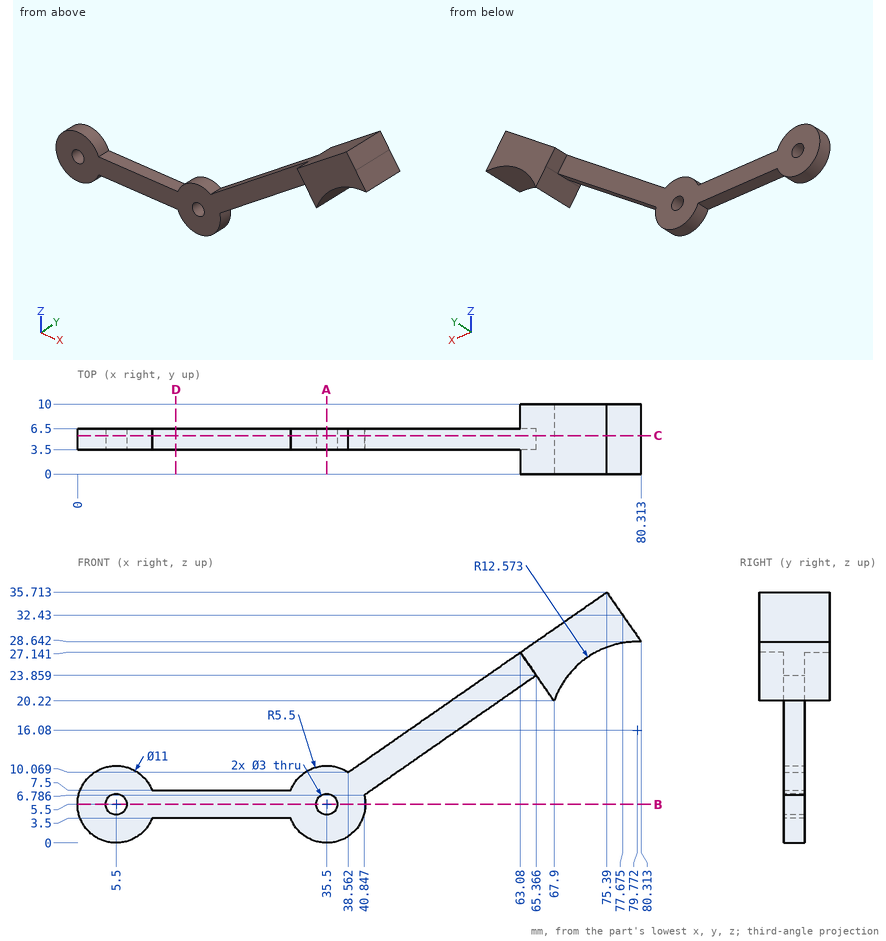
Input: dimensioned drawing with shaded views. Units: mm. Origin: part minimum x, y, z. Coordinates: 2 decimals unless noted, no trailing zeros. Loops run counter-clockwise (first coordinate to the right, second up) from the corner with the lowest first, then second, coordinate; pieces in that order, holes last. Notation, with made-up numbers: (-6, -40) - (27, -40) arc R19 ccw to (27, -13) - close; hole circle Ø7 at (75, 54). An arc over 180 degrees is marked (long way). One line per question, with ' | ' between items. Start each with the question number.
(1) Ray query, L1, parallel to Z at x = 35.5, y = 4.95; L2, parallel to Y at x = 56.5, z = 20; L3, parallel to Z at x = 16.5, y = 6.25. Return the intervals inside material, ascending. Write a range as from..to.
(2) Cut plane A-A on x = 35.5. Output: boundary loops of the cut face in (y, z).
(3) Cut plane D-D on x = 14. Output: boundary loops of the cut face in (y, z), and give its area (3 significant figures).
(4) Cut plane C-C on y = 5.5. Output: boundary loops of the cut face in (x, z) (1 decimal), and give its area (3 significant figures).
(5) First-contact query: pin 1 (0.9 mm diameter, centred on x = 16, y = 5.5, fed in from +Z); pin 2 (2.5 mm diameter, centred on x = 35.5, z = 5.5, fed in from -Y); pin 3 (5 mm diameter, centred on x = 30, y = 5, fed in from +Z); pin 4 (10 mm diameter, centred on x = 10, z = 11, fed in from -Y). Flat tips, straight axial feed; report the tip coordinate or a pass-through.
(6) Cut plane B-B on z = 5.5. Output: boundary loops of the cut face in (x, y), and give its area (3 significant figures).
Here are the results:
1) L1: 0..4, 7..11 | L2: 3.5..6.5 | L3: 3.5..7.5
2) outline: (3.5, 0) - (6.5, 0) - (6.5, 4) - (3.5, 4) - close; (3.5, 7) - (6.5, 7) - (6.5, 11) - (3.5, 11) - close
3) outline: (3.5, 3.5) - (6.5, 3.5) - (6.5, 7.5) - (3.5, 7.5) - close | area: 12.0 mm²
4) outline: (10.6, 3.5) - (30.4, 3.5) arc R5.5 ccw to (40.8, 6.8) - (65.4, 23.9) - (67.9, 20.2) arc R12.6 cw to (80.3, 28.6) - (75.4, 35.7) - (38.6, 10.1) arc R5.5 ccw to (30.4, 7.5) - (10.6, 7.5) arc R5.5 ccw (long way) to start; hole circle Ø3 at (5.5, 5.5); hole circle Ø3 at (35.5, 5.5) | area: 474 mm²
5) pin 1: z = 7.5 | pin 2: through | pin 3: z = 10.11 | pin 4: y = 3.5
6) outline: (0, 3.5) - (4, 3.5) - (4, 6.5) - (0, 6.5) - close; (7, 3.5) - (34, 3.5) - (34, 6.5) - (7, 6.5) - close; (37, 3.5) - (41, 3.5) - (41, 6.5) - (37, 6.5) - close | area: 105 mm²
